```python
from build123d import *

# Parameters (mm, degrees)
F0_R     = 15
F1_DEPTH = 4
F3_DEPTH = 25
F4_R     = 15


with BuildPart() as f1:
    # F0 (on Top) → F1 (new body)
    with BuildSketch(Plane.XY):
        with BuildLine():
            Line((84, 0), (0, 0))
            Line((0, 0), (0, -84))
            Line((0, -84), (42, -84))
            ThreePointArc((42, -84), (71.698485, -71.698485), (84, -42))
            Line((84, -42), (84, 0))
        make_face()
        with Locations((42, -42)):
            Circle(F0_R, mode=Mode.SUBTRACT)
    extrude(amount=F1_DEPTH)

    # F2 (on face) → F3 (join)
    with BuildSketch(Plane(origin=(0, 0, 0), x_dir=(1, 0, 0), z_dir=(0, 0, -1))):
        Polygon((84, 4), (4, 4), (4, 84), (0, 84), (0, 0), (84, 0), align=None)
    extrude(amount=F3_DEPTH)

    # F4
    f4_edges = [f1.edges().sort_by_distance(p)[0] for p in [
        (2, -84, -25),
        (84, -2, -25),
    ]]
    fillet(f4_edges, radius=F4_R)


solid = f1.part
```
The model under review builds one solid part; all positions refer to its coordinate system, in mm. A direction names the side the tool comes from. Round coordinates to 2 decimals unless told otherwise and drop trailing zeros. Loops run counter-clockwise (first coordinate to the right, second up) from the corner with the lowest first, then second, coordinate; pieces in that order, holes last. Notation, with made-up numbers: M 26.25,-8 L 74.25,-8 A28 ccw 74.25,13 Z; hole C -21,18.5 d2. An arc over 180 degrees is marked long. Answer as a JSON object with one key per item and string values.
(1) Take a section at D-D on z = -22.5. Give the boundary of the cut face in (x, y), and give its area (3 significant figures).
Resolved:
{"outline": "M 0,-77.29 L 4,-77.29 L 4,-4 L 77.29,-4 L 77.29,0 L 0,0 Z", "area": "602 mm²"}
(2) Clearance check with flat-ended pins moving along their axes: P1, Ø4, axis at x = 51.5, z = -8, coming from the +Y side; P2, Ø12, axis at x = 14.5, y = -50.5, coming from the -Z side; P3, Ø8, axis at x = 64.5, z = -20, coming from the -Y side; P4, Ø2, axis at y = -56, z = -18.5, coming from the +X side. State where each tip first meets the part, or that it passes through.
Resolved:
{"P1": "y = 0", "P2": "z = 0", "P3": "y = -4", "P4": "x = 4"}
(3) Draft analysis for pull direction X (two halves, no side actions). For faces 3 (the cylindrical face through (1.97, -79.49, -20.72)), 4 (the cylindrical face through (30.944, -31.862, 1.972)), 5 (the flat face through (4, -43, -12)), state which applies: released by +X, released by -X, zero draft, split by the parting line, or undercut.
Resolved:
{"face 3": "zero draft", "face 4": "undercut", "face 5": "released by +X"}
(4) Take a section at C-C on z = 2. Give the boundary of the cut face in (x, y), and give its area (3 significant figures).
Resolved:
{"outline": "M 0,-84 L 42,-84 A42 ccw 84,-42 L 84,0 L 0,0 Z; hole C 42,-42 d30", "area": "5,970 mm²"}
(5) To check wall thickness, follow line 1 along Y through (x, z) = (42, 2.3); line 2 along Z through (x, y) = (57.5, -6). State the ranges of each line that lie inside material, in increasing order.
Resolved:
{"line 1": "-84 to -57, -27 to 0", "line 2": "0 to 4"}
(6) Tool access review of faces 1 (the flat face through (43, -26, 0)), 2 (the cylindrical face through (71.37, -72.023, 1.972)): name each direction out of +Z, -Z, +X, -X, +Y, -Y from which nothing blocks a thin tool from reaching the whole face with its end or side.
Resolved:
{"face 1": "-Z, +X, -Y", "face 2": "+Z, -Z, +X, -Y"}
(7) Take a section at B-B on y = -24. Give the boundary of the cut face in (x, z), and give its area (3 significant figures).
Resolved:
{"outline": "M 0,-25 L 4,-25 L 4,0 L 84,0 L 84,4 L 0,4 Z", "area": "436 mm²"}
(8) Take a section at A-A on x = 30.5. Give the boundary of the cut face in (y, z).
Resolved:
{"outline": "M -84,0 L -51.63,0 L -51.63,4 L -84,4 Z; M -32.37,0 L -4,0 L -4,-25 L 0,-25 L 0,4 L -32.37,4 Z"}
